Could you check a few things on this model? Use its own coordinates, in mm. A direction names the side the tool comes from. Give positions to 0.01 mm unless a question says otherwise; leave off trailing zeros. Order: outer loops, then holes, each group sorted by start corner. A loop starts at its lowest first (then second) coordinate and runs counter-clockwise, first axis right, second up. Notation, with made-up numbers: (42, -37.75) - (48, -37.75) arc R5 cw to (48, -33.75) - close; hole circle Ø8 at (49, -27.75). An arc over 180 degrees is marked (long way). Put each result on its own line as item: value.
from build123d import *

# Parameters (mm, degrees)
SKETCH1_R           = 11.938
BOSS_EXTRUDE1_DEPTH = 25.4
SKETCH2_R           = 10.16
SKETCH2_R_2         = 2.54
CUT_EXTRUDE1_DEPTH  = 1.27
SKETCH3_R           = 1.5875
BOSS_EXTRUDE2_DEPTH = 38.1


with BuildPart() as part:
    # Sketch1 → Boss-Extrude1 (new body)
    with BuildSketch(Plane(origin=(0, 0, 0), x_dir=(1, 0, 0), z_dir=(0, 1, 0))):
        Circle(SKETCH1_R)
    extrude(amount=BOSS_EXTRUDE1_DEPTH)

    # Sketch2 → Cut-Extrude1 (cut)
    with BuildSketch(Plane(origin=(0, 25.4, 0), x_dir=(1, 0, 0), z_dir=(0, 1, 0))):
        Circle(SKETCH2_R)
        Circle(SKETCH2_R_2, mode=Mode.SUBTRACT)
    extrude(amount=-CUT_EXTRUDE1_DEPTH, mode=Mode.SUBTRACT)

    # Sketch3 → Boss-Extrude2 (add)
    with BuildSketch(Plane.XY):
        with Locations((0, 3.175)):
            Circle(SKETCH3_R)
    extrude(amount=BOSS_EXTRUDE2_DEPTH)


solid = part.part
1) Suppose I cut it at B-B, the plane x = 0. List the corners of the cut face in (y, z) for me.
Filled in:
outline: (0, -11.94) - (25.4, -11.94) - (25.4, -10.16) - (24.13, -10.16) - (24.13, -2.54) - (25.4, -2.54) - (25.4, 2.54) - (24.13, 2.54) - (24.13, 10.16) - (25.4, 10.16) - (25.4, 11.94) - (4.76, 11.94) - (4.76, 38.1) - (1.59, 38.1) - (1.59, 11.94) - (0, 11.94) - close
2) I'm going to push flat-ended pins straight in: pin 1 (10 mm diameter, centred on y = 16, z = 7, fed in from -X); pin 2 (10 mm diameter, centred on y = 10, z = 10.5, fed in from +X); pin 3 (10 mm diameter, centred on x = -5, z = 18, fed in from -Y); pin 4 (6 mm diameter, centred on x = 3.5, z = -1.5, fed in from +Y). Where does each tip first touch, or does it pass through?
Filled in:
pin 1: stops at x = -11.77
pin 2: stops at x = 10.6
pin 3: stops at y = 1.59
pin 4: stops at y = 25.4
3) If I drill on line 1 (Z direction, x = 0, y = 24.75); line 2 (Z direction, x = 1.75, y = 24.5), over which ranges is the centre line in solid material (lowest first)? Write a range as [from, to].
Filled in:
line 1: z = [-11.94, -10.16], [-2.54, 2.54], [10.16, 11.94]
line 2: z = [-11.81, -10.01], [-1.84, 1.84], [10.01, 11.81]
4) Suppose I cut it at D-D, the plane x = 7.75. List the corners of the cut face in (y, z) for me.
Filled in:
outline: (0, -9.08) - (25.4, -9.08) - (25.4, -6.57) - (24.13, -6.57) - (24.13, 6.57) - (25.4, 6.57) - (25.4, 9.08) - (0, 9.08) - close
5) Suppose I cut it at C-C, the plane y = 9.5. List the corners of the cut face in (x, z) for me, and give its area (3 significant figures).
Filled in:
outline: circle Ø23.88 at (0, 0)
area: 448 mm^2
6) We'd pull the mould along Z, two halves only. Please class faces 3 (the cylindrical face through (-0.33, 24.77, -2.52)), 4 (the cylindrical face through (0.853, 4.514, 24.78)), 5 (the cylindrical face through (-2.588, 12.522, 11.654)), 6 (the cylindrical face through (-1.323, 24.774, -10.074)): pulls with the +Z half, pulls with the -Z half, needs draft (parallel to the pull), parting line crosses it, or undercut.
Filled in:
face 3: undercut
face 4: needs draft
face 5: parting line crosses it
face 6: undercut
7) Suppose I cut it at A-A, the plane z = 0. List the corners of the cut face in (x, y) for me.
Filled in:
outline: (-11.94, 0) - (11.94, 0) - (11.94, 25.4) - (10.16, 25.4) - (10.16, 24.13) - (2.54, 24.13) - (2.54, 25.4) - (-2.54, 25.4) - (-2.54, 24.13) - (-10.16, 24.13) - (-10.16, 25.4) - (-11.94, 25.4) - close
8) Which directions (+Z, -Z, +X, -X, +Y, -Y) give clear straight access to the entire face, cutting with the end or side of a thin tool? Please do faces 1 (the flat face through (2, 24.13, 2)), 2 (the flat face through (0, 25.4, 0)).
Filled in:
face 1: +Y
face 2: +Z, -Z, +X, -X, +Y
